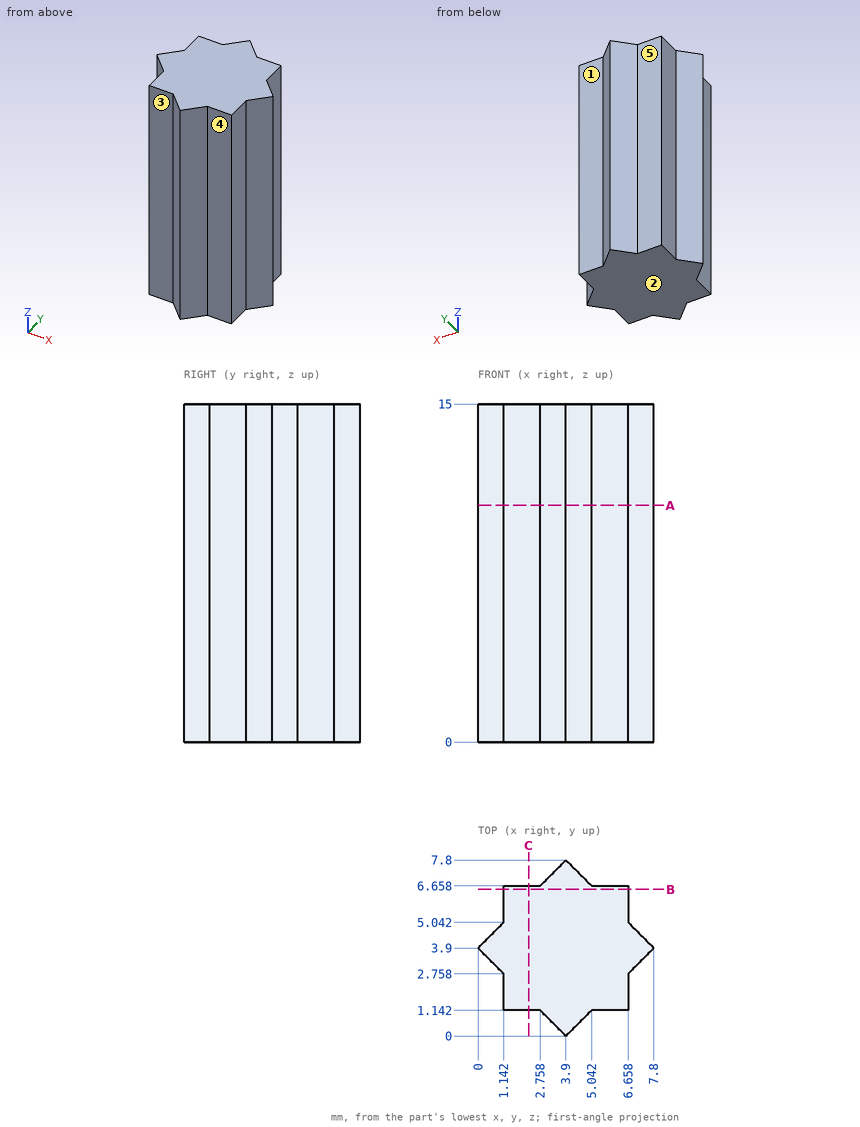
Part print with two shaded views. Sizes in mm from the minimum x, y, z corner. A direction names the side the tool comes from. Give positions to 0.01 mm unless a question says otherwise; leave off trailing zeros. Order: outer loops, then holes, each group sorted by start corner. A loop starts at its lowest first (then second) coordinate and runs counter-clockwise, first axis right, second up.
1) Wall check: probe 1 along X at (y, z) = (5.5, 8.25); probe 2 along Y at (x, z) = (0.75, 10.25). Give the ranges that are in metal, low to high.
2) Saw through at B-B, the plane y = 6.5. Write the cut outline in (x, z).
3) Saw through at A-A, the plane z = 10.5. Write the cut outline in (x, y).
4) Pin check, flat tips, straight feed: pin 1 (0.8 mm diameter, centred on y = 5.5, z = 5.5, fed in from -X); pin 2 (1.3 mm diameter, centred on y = 5.5, z = 5, fed in from +X); pin 3 (1.5 mm diameter, centred on x = 2.5, z = 3, fed in from -Y). Stop position of each tip, or through.
5) 3-axis set-ups, long thin cutter, end or side, ignore diameter. For the marked faces 1, 2, 3, 4 and 5: which of +Z, -Z, +X, -X, +Y, -Y reach the whole face in a straight line?
Computed:
1. probe 1: x = 1.14 to 6.66
1. probe 2: y = 3.15 to 4.65
2. outline: (1.14, 0) - (6.66, 0) - (6.66, 15) - (1.14, 15) - close
3. outline: (0, 3.9) - (1.14, 2.76) - (1.14, 1.14) - (2.76, 1.14) - (3.9, 0) - (5.04, 1.14) - (6.66, 1.14) - (6.66, 2.76) - (7.8, 3.9) - (6.66, 5.04) - (6.66, 6.66) - (5.04, 6.66) - (3.9, 7.8) - (2.76, 6.66) - (1.14, 6.66) - (1.14, 5.04) - close
4. pin 1: stops at x = 1.14
4. pin 2: stops at x = 6.85
4. pin 3: stops at y = 0.65
5. face 1: +Z, -Z, +X, +Y
5. face 2: -Z, +X, -X, +Y, -Y
5. face 3: +Z, -Z, -X, -Y
5. face 4: +Z, -Z, +X, -Y
5. face 5: +Z, -Z, -X, +Y
